Source: CAD feature listing. Evaluate the final solid. Frame: model axes, mm. Face numbers are marked on the shaded views. A direction names the side the tool comes from. Coordinates: 2 decimals unless noted, no trailing zeros. Loops run counter-clockwise (first coordinate to the right, second up) from the corner with the lowest first, then second, coordinate; pieces in that order, holes last. Notation, with made-up numbers: (51, 37) -> (91, 37) arc R17 cw to (91, 45) -> close; hole circle Ø10 at (-30, -38). An arc over 180 degrees is marked (long way). Answer as a JSON object with one key per item and string values. Group by question number.
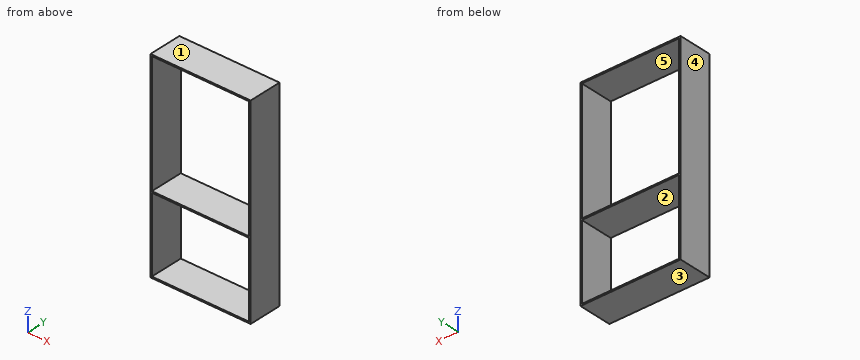
from build123d import *

# Parameters (mm, degrees)
F0_W     = 889
F0_H     = 12.7
F1_DEPTH = 304.8


with BuildPart() as f1:
    # F0 (on Front) → F1 (new body)
    with BuildSketch(Plane.XZ):
        with Locations((-161.960473, 895.35)):
            Rectangle(F0_W, F0_H)
        Polygon((-606.460473, 889), (-606.460473, 901.7), (-619.160473, 901.7), (-619.160473, -927.1), (-606.460473, -927.1), (-606.460473, -914.4), (-606.460473, -609.6), (-606.460473, -596.9), (-606.460473, -419.1), (-606.460473, -406.4), (-606.460473, -228.6), (-606.460473, -215.9), (-606.460473, -63.5), (-606.460473, -50.8), (-606.460473, 76.2), (-606.460473, 88.9), (-606.460473, 215.9), (-606.460473, 228.6), (-606.460473, 304.8), (-606.460473, 317.5), (-606.460473, 393.7), (-606.460473, 406.4), (-606.460473, 469.9), (-606.460473, 482.6), align=None)
        Polygon((295.239527, 901.7), (282.539527, 901.7), (282.539527, 889), (282.539527, 482.6), (282.539527, 469.9), (282.539527, -215.9), (282.539527, -228.6), (282.539527, -406.4), (282.539527, -419.1), (282.539527, -596.9), (282.539527, -609.6), (282.539527, -914.4), (282.539527, -927.1), (295.239527, -927.1), align=None)
        with Locations((-161.960473, -920.75)):
            Rectangle(F0_W, F0_H)
        Polygon((282.539527, -228.6), (282.539527, -215.9), (257.139527, -215.9), (-200.060473, -215.9), (-225.460473, -215.9), (-238.160473, -215.9), (-606.460473, -215.9), (-606.460473, -228.6), align=None)
    extrude(amount=F1_DEPTH)


solid = f1.part
1. Reachability of the marked faces 1 and 2 from +Z, -Z, +X, -X, +Y, -Y: full face, straight path, thin tool, end or side. Return the list, or none.
2. Section query C-C on x = -413.5. Return loops of the section in (y, z), then the cut area to 3 significant figures.
3. Ray query, L1, parallel to Z at x = 160, y = -177.5; L2, parallel to X at y = -262, z = -841.5. Return the intervals inside material, ascending.
4. Mould query, pull axis Z, two halves, no side actions, for the marked faces 3, 4 and 5. Classes: pulls with the +Z half, pulls with the -Z half, needs draft (parallel to the pull), parting line crosses it, or undercut.
5. Section query A-A on y = -254. Return loops of the section in (x, z), then the cut area to 3 significant figures.
6. Section query B-B on z = 572.5. Return loops of the section in (x, y), then the cut area to 3 significant figures.
Solved:
{
 "1": {"face 1": "+Z, +X, -X, +Y, -Y", "face 2": "+Y, -Y"},
 "2": {"outline": "(-304.8, -927.1) -> (0, -927.1) -> (0, -914.4) -> (-304.8, -914.4) -> close; (-304.8, -228.6) -> (0, -228.6) -> (0, -215.9) -> (-304.8, -215.9) -> close; (-304.8, 889) -> (0, 889) -> (0, 901.7) -> (-304.8, 901.7) -> close", "area": "11,600 mm^2"},
 "3": {"L1": "-927.1 to -914.4, -228.6 to -215.9, 889 to 901.7", "L2": "-619.16 to -606.46, 282.54 to 295.24"},
 "4": {"face 3": "pulls with the -Z half", "face 4": "needs draft", "face 5": "undercut"},
 "5": {"outline": "(-619.16, -927.1) -> (295.24, -927.1) -> (295.24, 901.7) -> (-619.16, 901.7) -> close; hole (-606.46, -914.4) -> (282.54, -914.4) -> (282.54, -228.6) -> (-606.46, -228.6) -> close; hole (-606.46, -215.9) -> (282.54, -215.9) -> (282.54, 889) -> (-606.46, 889) -> close", "area": "80,300 mm^2"},
 "6": {"outline": "(-619.16, -304.8) -> (-606.46, -304.8) -> (-606.46, 0) -> (-619.16, 0) -> close; (282.54, -304.8) -> (295.24, -304.8) -> (295.24, 0) -> (282.54, 0) -> close", "area": "7,740 mm^2"}
}
